from build123d import *

# Parameters (mm, degrees)
F2_DEPTH      = 6.5
F2_DEPTH_BACK = 1.5
F3_W          = 2
F3_H          = 5.2
F4_DEPTH      = 5.95
F5_W          = 13
F5_H          = 3
F6_DEPTH      = 12.5
F7_R          = 1.25
F8_DEPTH      = 10


with BuildPart() as f2:
    # F1 (on Top) → F2 (new body, two sides)
    with BuildSketch(Plane.XY) as f2_sk:
        with BuildLine():
            ThreePointArc((20.5, 5.5), (19.0355339059, 9.0355339059), (15.5, 10.5))
            Line((15.5, 10.5), (-15.5, 10.5))
            ThreePointArc((-15.5, 10.5), (-19.0355339059, 9.0355339059), (-20.5, 5.5))
            Line((-20.5, 5.5), (-20.5, -5.5))
            ThreePointArc((-20.5, -5.5), (-19.0355339059, -9.0355339059), (-15.5, -10.5))
            Line((-15.5, -10.5), (15.5, -10.5))
            ThreePointArc((15.5, -10.5), (19.0355339059, -9.0355339059), (20.5, -5.5))
            Line((20.5, -5.5), (20.5, 5.5))
        make_face()
    extrude(amount=F2_DEPTH)
    extrude(f2_sk.sketch, amount=-F2_DEPTH_BACK)

    # F3 (on Front) → F4 (cut, symmetric)
    with BuildSketch(Plane.XZ):
        with BuildLine():
            ThreePointArc((3.6728735344, -2.6), (4.2882357039, -1.3641974005), (4.5, 0))
            ThreePointArc((4.5, 0), (4.2882357039, 1.3641974005), (3.6728735344, 2.6))
            Line((3.6728735344, 2.6), (-3.6728735344, 2.6))
            ThreePointArc((-3.6728735344, 2.6), (-4.5, 0), (-3.6728735344, -2.6))
            Line((-3.6728735344, -2.6), (3.6728735344, -2.6))
        make_face()
        with BuildLine():
            ThreePointArc((3.6728735344, 2.6), (4.2882357039, 1.3641974005), (4.5, 0))
            ThreePointArc((4.5, 0), (4.2882357039, -1.3641974005), (3.6728735344, -2.6))
            Line((3.6728735344, -2.6), (8, -2.6))
            Line((8, -2.6), (8, 2.6))
            Line((8, 2.6), (3.6728735344, 2.6))
        make_face()
        with BuildLine():
            Line((-3.6728735344, 2.6), (3.6728735344, 2.6))
            ThreePointArc((3.6728735344, 2.6), (0, 4.5), (-3.6728735344, 2.6))
        make_face()
        with BuildLine():
            ThreePointArc((-3.6728735344, -2.6), (0, -4.5), (3.6728735344, -2.6))
            Line((3.6728735344, -2.6), (-3.6728735344, -2.6))
        make_face()
        with BuildLine():
            ThreePointArc((-3.6728735344, -2.6), (-4.5, 0), (-3.6728735344, 2.6))
            Line((-3.6728735344, 2.6), (-8, 2.6))
            Line((-8, 2.6), (-8, -2.6))
            Line((-8, -2.6), (-3.6728735344, -2.6))
        make_face()
        with Locations((-9, 0)):
            Rectangle(F3_W, F3_H)
    extrude(amount=F4_DEPTH, both=True, mode=Mode.SUBTRACT)

    # F5 (on Front) → F6 (cut, symmetric)
    with BuildSketch(Plane.XZ):
        Rectangle(F5_W, F5_H)
    extrude(amount=F6_DEPTH, both=True, mode=Mode.SUBTRACT)

    # F7 (on face) → F8 (cut)
    with BuildSketch(Plane(origin=(0, 0, -1.5), x_dir=(1, 0, 0), z_dir=(0, 0, -1))):
        with Locations((-12.5, 0)):
            Circle(F7_R)
        with Locations((12.5, 0)):
            Circle(F7_R)
    extrude(amount=-F8_DEPTH, mode=Mode.SUBTRACT)


solid = f2.part
Geometry check sheet. Reference: the model listing, model coordinates, mm. A direction names the side the tool comes from. Give positions to 0.01 mm unless a question says otherwise; leave off trailing zeros. Order: outer loops, then holes, each group sorted by start corner. A loop starts at its lowest first (then second) coordinate and runs counter-clockwise, first axis right, second up.
1. Sectioned sample at D-D (z = 3.75). Record the boundary of the cut face in (x, y), then the cut area to 3 significant figures.
Completed:
outline: (-20.5, -5.5) arc R5 ccw to (-15.5, -10.5) - (15.5, -10.5) arc R5 ccw to (20.5, -5.5) - (20.5, 5.5) arc R5 ccw to (15.5, 10.5) - (-15.5, 10.5) arc R5 ccw to (-20.5, 5.5) - close; hole circle Ø2.5 at (-12.5, 0); hole (-2.49, -5.95) - (2.49, -5.95) - (2.49, 5.95) - (-2.49, 5.95) - close; hole circle Ø2.5 at (12.5, 0)
area: 771 mm2
2. Sectioned sample at B-B (x = -12.5). Record the boundary of the cut face in (y, z).
Completed:
outline: (-10.5, -1.5) - (-1.25, -1.5) - (-1.25, 6.5) - (-10.5, 6.5) - close; (1.25, -1.5) - (10.5, -1.5) - (10.5, 6.5) - (1.25, 6.5) - close
3. Access from +Z, -Z, +X, -X, +Y, -Y to the whole of each face (thin tool, end or side, straight path). Record for faces 4 (the face through (6, 0, 2.6)), 5 (the face through (-6.5, 8, 0)), 6 (the face through (0, 10.5, 3)).
Completed:
face 4: -Z
face 5: -Z, +Y, -Y
face 6: +Z, -Z, +X, -X, +Y
4. Sectioned sample at C-C (y = 0). Record the boundary of the cut face in (x, z), then the cut area to 3 significant figures.
Completed:
outline: (-20.5, -1.5) - (-13.75, -1.5) - (-13.75, 6.5) - (-20.5, 6.5) - close; (-11.25, -1.5) - (-10, -1.5) - (-10, 2.6) - (-3.67, 2.6) arc R4.5 cw to (3.67, 2.6) - (8, 2.6) - (8, -1.5) - (11.25, -1.5) - (11.25, 6.5) - (-11.25, 6.5) - close; (13.75, -1.5) - (20.5, -1.5) - (20.5, 6.5) - (13.75, 6.5) - close
area: 204 mm2
5. Draft check along X on faces 1 (the face through (-10, 0, 1)), 2 (the face through (0, 0, 6.5)), 3 (the face through (19.07, 9, 2.56)). Enter one of: pulls with the +X half, pulls with the -X half, needs draft (parallel to the pull), parting line crosses it, or undercut.
Completed:
face 1: undercut
face 2: needs draft
face 3: pulls with the +X half
6. Scan lines: line 1 (X direction, y = 0, z = 5.25); line 2 (X direction, y = 0, z = 1.5); line 3 (Y direction, x = 12.5, z = 2.25). Record each from-to range of solid material in increasing order.
Completed:
line 1: x = -20.5 to -13.75, -11.25 to 11.25, 13.75 to 20.5
line 2: x = -20.5 to -13.75, -11.25 to -10, 8 to 11.25, 13.75 to 20.5
line 3: y = -10.5 to -1.25, 1.25 to 10.5
7. Depth check by flat-ended pin: pin 1 (3.5 mm diameter, centred on x = 2, y = 7, fed in from -Z); pin 2 (2 mm diameter, centred on x = -12.5, y = 0, fed in from -Z); pin 3 (0.9 mm diameter, centred on y = 9, z = -0.5, fed in from -X); pin 4 (3.5 mm diameter, centred on y = -9, z = 0, fed in from -X). Enter the tip coordinate at first touch or a pass-through.
Completed:
pin 1: stops at z = 1.5
pin 2: passes through
pin 3: stops at x = -19.46
pin 4: stops at x = -20.18
8. Sectioned sample at A-A (z = 1). Record the boundary of the cut face in (x, y), then the cut area to 3 significant figures.
Completed:
outline: (-20.5, -5.5) arc R5 ccw to (-15.5, -10.5) - (-6.5, -10.5) - (-6.5, -5.95) - (-10, -5.95) - (-10, 5.95) - (-6.5, 5.95) - (-6.5, 10.5) - (-15.5, 10.5) arc R5 ccw to (-20.5, 5.5) - close; (6.5, -10.5) - (15.5, -10.5) arc R5 ccw to (20.5, -5.5) - (20.5, 5.5) arc R5 ccw to (15.5, 10.5) - (6.5, 10.5) - (6.5, 5.95) - (8, 5.95) - (8, -5.95) - (6.5, -5.95) - close; hole circle Ø2.5 at (-12.5, 0); hole circle Ø2.5 at (12.5, 0)
area: 497 mm2
